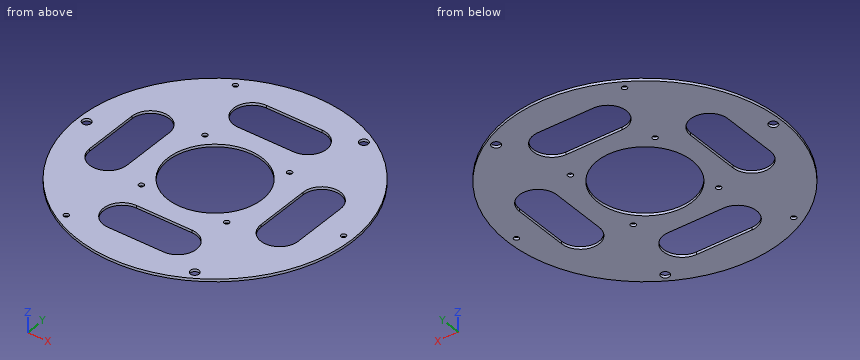
from build123d import *

# Parameters (mm, degrees)
CROQUIS1_R              = 160
CROQUIS1_R_2            = 55
CROQUIS1_R_3            = 5.1
CROQUIS1_R_4            = 3
SALIENTE_EXTRUIR2_DEPTH = 3


with BuildPart() as part:
    # Croquis1 → Saliente-Extruir2 (new body)
    with BuildSketch(Plane.XY):
        Circle(CROQUIS1_R)
        Circle(CROQUIS1_R_2, mode=Mode.SUBTRACT)
        with Locations((-150, 0)):
            Circle(CROQUIS1_R_3, mode=Mode.SUBTRACT)
        with Locations((-48.532730183, -49.522943911)):
            Circle(CROQUIS1_R_4, mode=Mode.SUBTRACT)
        with Locations((75, 129.903810568)):
            Circle(CROQUIS1_R_3, mode=Mode.SUBTRACT)
        with Locations((75, -129.903810568)):
            Circle(CROQUIS1_R_3, mode=Mode.SUBTRACT)
        with Locations((-75, 129.903810568)):
            Circle(CROQUIS1_R_4, mode=Mode.SUBTRACT)
        with Locations((150, 0)):
            Circle(CROQUIS1_R_4, mode=Mode.SUBTRACT)
        with Locations((-75, -129.903810568)):
            Circle(CROQUIS1_R_4, mode=Mode.SUBTRACT)
        with Locations((-49.499768998, 49.495180262)):
            Circle(CROQUIS1_R_4, mode=Mode.SUBTRACT)
        with Locations((50.43565577, -48.541164253)):
            Circle(CROQUIS1_R_4, mode=Mode.SUBTRACT)
        with Locations((49.144383708, 49.848064656)):
            Circle(CROQUIS1_R_4, mode=Mode.SUBTRACT)
        with BuildLine():
            Line((-32.5, 78.157247055), (32.5, 78.157247055))
            ThreePointArc((32.5, 78.157247055), (54.279441944, 100), (32.5, 121.842752945))
            Line((32.5, 121.842752945), (-32.5, 121.842752945))
            ThreePointArc((-32.5, 121.842752945), (-54.342752945, 100), (-32.5, 78.157247055))
        make_face(mode=Mode.SUBTRACT)
        with BuildLine():
            Line((-32.5, -121.842752945), (32.5, -121.842752945))
            ThreePointArc((32.5, -121.842752945), (54.279441944, -100), (32.5, -78.157247055))
            Line((32.5, -78.157247055), (-32.5, -78.157247055))
            ThreePointArc((-32.5, -78.157247055), (-54.342752945, -100), (-32.5, -121.842752945))
        make_face(mode=Mode.SUBTRACT)
        with BuildLine():
            Line((78.157247055, 32.5), (78.157247055, -32.5))
            ThreePointArc((78.157247055, -32.5), (100, -54.342752945), (121.842752945, -32.5))
            Line((121.842752945, -32.5), (121.842752945, 32.5))
            ThreePointArc((121.842752945, 32.5), (100, 54.342752945), (78.157247055, 32.5))
        make_face(mode=Mode.SUBTRACT)
        with BuildLine():
            Line((-78.157247055, 32.5), (-78.157247055, -32.5))
            ThreePointArc((-78.157247055, -32.5), (-100, -54.342752945), (-121.842752945, -32.5))
            Line((-121.842752945, -32.5), (-121.842752945, 32.5))
            ThreePointArc((-121.842752945, 32.5), (-100, 54.342752945), (-78.157247055, 32.5))
        make_face(mode=Mode.SUBTRACT)
    extrude(amount=SALIENTE_EXTRUIR2_DEPTH)


solid = part.part
Verification items for the finished model (mm, model axes). Coordinates: 2 decimals unless noted, no trailing zeros. Order: outer loops, then holes, each group sorted by start corner. A loop starts at its lowest first (then second) coordinate and runs counter-clockwise, first axis right, second up. Notation, with made-up numbers: M 79,33.25 L 121,33.25 A20 cw 121,48.25 Z; hole C -2.75,-37.75 d10. An arc over 180 degrees is marked long. One line per item, written item: value. Start each with the question number.
Item 1: Depth check by flat-ended pin: P1, Ø1.5, axis at x = -121.5, z = 1, coming from the -Y side. Enter the tip coordinate at first touch or a pass-through.
Item 2: Sectioned sample at D-D on z = 0.55. Give the number of separate pieces and of enclosed holes in the cut face, then the cut area to 3 significant figures.
Item 3: Sectioned sample at B-B on y = 94.5. Record the cut outline in (x, z).
Item 4: Thickness scan on probe 1 along Y at (x, z) = (72, 1.45); probe 2 along Y at (x, z) = (-75, 2.05); probe 3 along Y at (x, z) = (-13, 1.05). Record the ranges inside material, lowest first.
Item 5: Sectioned sample at C-C on x = 100. Record the cut outline in (y, z), then the cut area to 3 significant figures.
Item 6: Sectioned sample at A-A on x = 13.5. Record the cut outline in (y, z).
Calculated:
1. P1: y = -104.97
2. separate pieces: 1
2. enclosed holes: 15
2. area: 53,100 mm^2
3. outline: M -129.11,0 L -53.64,0 L -53.64,3 L -129.11,3 Z; M 53.58,0 L 129.11,0 L 129.11,3 L 53.58,3 Z
4. probe 1: -142.88 to -134.03, -125.78 to 125.78, 134.03 to 142.88
4. probe 2: -141.33 to -132.9, -126.9 to 126.9, 132.9 to 141.33
4. probe 3: -159.47 to -121.84, -78.16 to -53.44, 53.44 to 78.16, 121.84 to 159.47
5. outline: M -124.9,0 L -54.34,0 L -54.34,3 L -124.9,3 Z; M 54.34,0 L 124.9,0 L 124.9,3 L 54.34,3 Z
5. area: 423 mm^2
6. outline: M -159.43,0 L -121.84,0 L -121.84,3 L -159.43,3 Z; M -78.16,0 L -53.32,0 L -53.32,3 L -78.16,3 Z; M 53.32,0 L 78.16,0 L 78.16,3 L 53.32,3 Z; M 121.84,0 L 159.43,0 L 159.43,3 L 121.84,3 Z
